CAD build for the part. Positions are in the model's coordinates, mm. A direction names the side the tool comes from. Round coordinates to 2 decimals unless told otherwise and drop trailing zeros. Order: outer loops, then holes, each group sorted by start corner. A loop starts at its lowest first (then second) coordinate and runs counter-clockwise, first axis right, second up. Notation, with made-up numbers: M 16,0 L 64,0 A26 ccw 64,23 Z; hole C 36,-21 d9. An arc over 180 degrees is marked long. Put each result on its own line as item: value.
Autodesk Inventor part; units mm, degrees
ref_plane "YZ Plane" through (0, 0, 0) normal (1, 0, 0) x (0, 1, 0)
ref_plane "XZ Plane" through (0, 0, 0) normal (0, 1, 0) x (-1, 0, 0)
ref_plane "XY Plane" through (0, 0, 0) normal (0, 0, 1) x (1, 0, 0)
sketch "Sketch1" plane through (0, 0, 0) normal (0, 1, 0) x (-1, 0, 0)
  circle A0 centre (0, 0) radius 7.75
  circle A1 centre (0, 0) radius 9.75
  dimension "d0" = 15.5
  dimension "d1" = 19.5
extrude "Extrusion1" add sketch "Sketch1" along normal blind 7
sketch "Sketch5" plane through (0, 7, 0) normal (0, 1, 0) x (1, 0, 0)
  circle A0 centre (0, 0) radius 11
  circle A1 centre (0, 0) radius 9
  dimension "d13" = 22
  dimension "d14" = 18
extrude "Extrusion5" add sketch "Sketch5" along normal blind 4
move faces "Move1" translate (0, 0.5, 0) faces at (8.4211, 7, 1.3362)
properties part number "685ZZFlanged_Adapter"
Item 1: Probe line 1 along Z through (x, y) = (0, 9.8); line 2 along Z through (x, y) = (0, 3.5); line 3 along Y through (x, z) = (-8, 2). List the from-to ranges inside material, lowest first. Write a range as [from, to].
Answers below:
line 1: [-11, -9], [9, 11]
line 2: [-9.75, -7.75], [7.75, 9.75]
line 3: [0, 7.5]
Item 2: Band-saw the part on B-B on z = 0. Give the cut face in (x, y).
Answers below:
outline: M -11,7 L -9.75,7 L -9.75,0 L -7.75,0 L -7.75,7.5 L -9,7.5 L -9,11 L -11,11 Z; M 7.75,0 L 9.75,0 L 9.75,7 L 11,7 L 11,11 L 9,11 L 9,7.5 L 7.75,7.5 Z
Item 3: Band-saw the part on A-A on x = 0. Give the cut face in (y, z), and give its area (4 significant figures).
Answers below:
outline: M 0,-9.75 L 7,-9.75 L 7,-11 L 11,-11 L 11,-9 L 7.5,-9 L 7.5,-7.75 L 0,-7.75 Z; M 0,7.75 L 7.5,7.75 L 7.5,9 L 11,9 L 11,11 L 7,11 L 7,9.75 L 0,9.75 Z
area: 45.25 mm²
Item 4: Tool access for faces 1 (the flat face through (-4, 7.5, 7)), 2 (the flat face through (7, 0, -4)): list every direction of +Z, -Z, +X, -X, +Y, -Y with a clear straight run to the whole face (end or side of a thin tool).
Answers below:
face 1: +Y
face 2: +Z, -Z, +X, -X, -Y
Item 5: Band-saw the part on C-C on y = 4. Give the cut face in (x, z), and give its area (3 significant figures).
Answers below:
outline: C 0,0 d19.5; hole C 0,0 d15.5
area: 110 mm²
Item 6: Pin check, flat tips, straight feed: P1, Ø3, axis at x = 3.5, y = 2.5, coming from the +Z side; P2, Ø1.5, axis at x = -6, y = 10, coming from the -Z side; P3, Ø1.5, axis at y = 8.5, z = -8.5, coming from the +X side. Stop position of each tip, or through.
Answers below:
P1: z = 9.54
P2: z = -9.67
P3: x = 7.81
Item 7: Mould opens along Z. For faces 3 (the cylindrical face through (-1.172, 9.226, 8.923)), 4 (the cylindrical face through (1.009, 3.698, -7.684)), 5 (the cylindrical face through (1.269, 3.451, -9.667)), 6 (the flat face through (-1, 7, 10)) say: pulls with the +Z half, pulls with the -Z half, needs draft (parallel to the pull), parting line crosses it, or undercut.
Answers below:
face 3: undercut
face 4: undercut
face 5: parting line crosses it
face 6: needs draft
Item 8: Band-saw the part on D-D on y = 10.25. Give the cut face in (x, z), and give its area (3 significant figures).
Answers below:
outline: C 0,0 d22; hole C 0,0 d18
area: 126 mm²
